from build123d import *

# Parameters (mm, degrees)
BASE_FLANGE1_DEPTH = 54
SKETCH6_R          = 1.984375
CUT_EXTRUDE1_DEPTH = 56.283583274


# Sheet-metal steps are written as plain solids
with BuildPart() as part:
    # Sketch1 → Base-Flange1 (new body)
    with BuildSketch(Plane(origin=(0, 0, 0), x_dir=(0, 0, -1), z_dir=(1, 0, 0))):
        with BuildLine():
            Line((-10, 0), (9.2634, 0))
            ThreePointArc((9.2634, 0), (9.784254855, 0.215745145), (10, 0.7366))
            Line((10, 0.7366), (10, 5))
            Line((10, 5), (10.7366, 5))
            Line((10.7366, 5), (10.7366, 0.7366))
            ThreePointArc((10.7366, 0.7366), (10.30510971, -0.30510971), (9.2634, -0.7366))
            Line((9.2634, -0.7366), (-10, -0.7366))
            Line((-10, -0.7366), (-10, 0))
        make_face()
    extrude(amount=BASE_FLANGE1_DEPTH)

    # Sketch6 → Cut-Extrude1 (cut, through all)
    with BuildSketch(Plane(origin=(0, 0, 0), x_dir=(1, 0, 0), z_dir=(0, 1, 0))):
        with Locations(Location((7.5, -0.7366, 0), (0, 0, 270))):
            Circle(SKETCH6_R)
        with Locations(Location((46.5, -0.7366, 0), (0, 0, 270))):
            Circle(SKETCH6_R)
    extrude(amount=-CUT_EXTRUDE1_DEPTH, mode=Mode.SUBTRACT)


solid = part.part
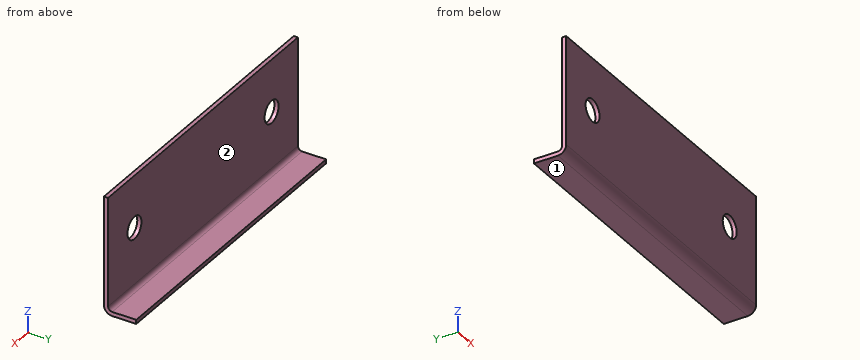
Read the model definition and answer for the solid it produces. Units are mm, in the model's axes. Face numbers are marked on the shaded views. A direction names the side the tool comes from. Give positions to 0.01 mm unless a question says otherwise; leave off trailing zeros. Write each loop counter-clockwise with the first axis right and the second up, starting at its lowest first coordinate (ties: lowest second). Pieces come first, ordered by that corner, then holes. Notation, with made-up numbers: M 39,18.25 L 61,18.25 A19 cw 61,51.25 Z; hole C 46.25,18.25 d4. An arc over 180 degrees is marked long. One line per item, written item: value. Start each with the question number.
(1) A flat-ended cylindrical pin translates along its axis: pin 1 Ø3 at (x, z) = (41, 2.5) entering from +Y. Find the tip coordinate at first contact, or state that the pin passes through.
(2) Find section C-C (z = -4.25). Determine the outline of the cut face in (x, y), plus the area to 3 significant figures.
(3) Find section D-D (y = 1.3). Determine the outline of the cut face in (x, z).
(4) Find section B-B (x = 46.5). Determine the outline of the cut face in (y, z), plus the area to 3 significant figures.
(5) Find section A-A (x = 4.5). Determine the outline of the cut face in (y, z), plus the area to 3 significant figures.
(6) A tool of negligible diameter and unlimited length cuts with its end or side. For the marked faces 1 and 2, from which of +Z, -Z, +X, -X, +Y, -Y can it reach the whole face along a straight path? Write none if from no direction.
(7) Find the intervals of material crossed by line 1 (Y direction, x = 37, z = -8); line 2 (Z direction, x = 14.5, y = 2.5); line 3 (Z direction, x = 50.5, y = -0.5), in increasing order.
Results below:
1. pin 1: stops at y = 0
2. outline: M 0,-0.74 L 54,-0.74 L 54,0 L 0,0 Z
2. area: 39.8 mm^2
3. outline: M 0,-10.74 L 54,-10.74 L 54,-10 L 0,-10 Z
4. outline: M -0.74,-9.26 A1.47 ccw 0.74,-10.74 L 5,-10.74 L 5,-10 L 0.74,-10 A0.74 cw 0,-9.26 L 0,-1.25 L -0.74,-1.25 Z; M -0.74,2.72 L 0,2.72 L 0,10 L -0.74,10 Z
4. area: 15.7 mm^2
5. outline: M -0.74,-9.26 A1.47 ccw 0.74,-10.74 L 5,-10.74 L 5,-10 L 0.74,-10 A0.74 cw 0,-9.26 L 0,10 L -0.74,10 Z
5. area: 18.6 mm^2
6. face 1: -Z, +X, -X, +Y, -Y
6. face 2: +Z, +X, -X, +Y
7. line 1: y = -0.74 to 0
7. line 2: z = -10.74 to -10
7. line 3: z = -10.06 to 10
